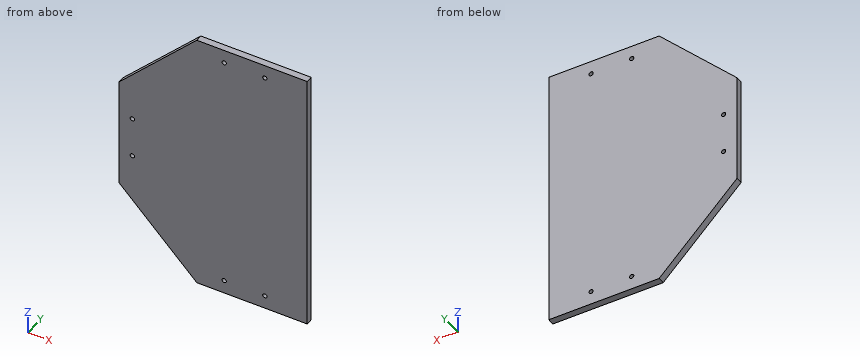
from build123d import *

# Parameters (mm, degrees)
BOSS_EXTRUDE1_DEPTH = 6.35
SKETCH2_R           = 1.995
CUT_EXTRUDE1_DEPTH  = 177.890707783
SKETCH5_R           = 1.995
CUT_EXTRUDE5_DEPTH  = 177.890707783
CUT_EXTRUDE6_DEPTH  = 10


with BuildPart() as part:
    # Sketch1 → Boss-Extrude1 (new body)
    with BuildSketch(Plane(origin=(0, 0, 0), x_dir=(1, 0, 0), z_dir=(0, 1, 0))):
        Polygon((125, 51.776695297), (51.776695297, 125), (-51.776695297, 125), (-125, 51.776695297), (-125, -51.776695297), (-51.776695297, -125), (51.776695297, -125), (125, -51.776695297), align=None)
    extrude(amount=BOSS_EXTRUDE1_DEPTH)

    # Sketch2 → Cut-Extrude1 (cut, through all)
    with BuildSketch(Plane(origin=(0, 6.35, 0), x_dir=(1, 0, 0), z_dir=(0, 1, 0))):
        with Locations(Location((-26.05, -112.3, 0), (0, 0, 270))):
            Circle(SKETCH2_R)
        with Locations(Location((12.05, -112.3, 0), (0, 0, 270))):
            Circle(SKETCH2_R)
        with Locations(Location((12.05, 112.3, 0), (0, 0, 90))):
            Circle(SKETCH2_R)
        with Locations(Location((-26.05, 112.3, 0), (0, 0, 90))):
            Circle(SKETCH2_R)
    extrude(amount=-CUT_EXTRUDE1_DEPTH, mode=Mode.SUBTRACT)

    # Sketch5 → Cut-Extrude5 (cut, through all)
    with BuildSketch(Plane(origin=(0, 6.35, 0), x_dir=(1, 0, 0), z_dir=(0, 1, 0))):
        with Locations(Location((-112.3, 19.05, 0), (0, 0, 270))):
            Circle(SKETCH5_R)
        with Locations(Location((-112.3, -19.05, 0), (0, 0, 270))):
            Circle(SKETCH5_R)
    extrude(amount=-CUT_EXTRUDE5_DEPTH, mode=Mode.SUBTRACT)

    # Sketch6 → Cut-Extrude6 (cut)
    with BuildSketch(Plane(origin=(0, 6.35, 0), x_dir=(1, 0, 0), z_dir=(0, 1, 0))):
        Polygon((51.776695297, -125), (125, -51.776695297), (125, 51.776695297), (51.776695297, 125), align=None)
    extrude(amount=-CUT_EXTRUDE6_DEPTH, mode=Mode.SUBTRACT)


solid = part.part
For this review, take the finished solid that the model builds, in its own axes (mm). Round coordinates to 2 decimals unless told otherwise and drop trailing zeros. Write each loop counter-clockwise with the first axis right and the second up, starting at its lowest first coordinate (ties: lowest second). Pieces come first, ordered by that corner, then holes. Notation, with made-up numbers: M 39,-23.75 L 71,-23.75 A20 cw 71,-7.75 Z; hole C -21.75,-8 d1. An arc over 180 degrees is marked long. Write item = value, one per line. Start each with the question number.
(1) Clearance check with flat-ended pins moving along their axes: pin 1 Ø4.5 at (x, z) = (12.05, -112.3) entering from +Y; pin 2 Ø2.5 at (x, z) = (-26.05, -112.3) entering from +Y; pin 3 Ø3 at (y, z) = (1, -73) entering from -X; pin 4 Ø3 at (y, z) = (2, -93) entering from -X. State where each tip first meets the part, or that it passes through.
(2) We need section B-B (z = 89). Give the boundary of the cut face in (x, y).
(3) We need section C-C (x = -86.5). Give the boundary of the cut face in (y, z).
(4) For line 1 along X through (y, z) = (3, -112.3) (3 decimals); line 2 along X through (y, z) = (1.5, 19.05) (3 decimals); line 3 along Z through (x, y) = (-114, 3.25), list the stretches that pass through material, from the lowest coordinate up.
(5) We need section A-A (y = 5). Give the boundary of the cut face in (x, z) (3 decimals), then the cut area to 3 significant figures.
Results found:
q1.pin_1 = 6.35
q1.pin_2 = through
q1.pin_3 = -105.28
q1.pin_4 = -85.28
q2.outline = M -87.78,0 L 51.78,0 L 51.78,6.35 L -87.78,6.35 Z
q3.outline = M 0,-90.28 L 6.35,-90.28 L 6.35,90.28 L 0,90.28 Z
q4.line_1 = -64.477 to -28.045, -24.055 to 10.055, 14.045 to 51.777
q4.line_2 = -125 to -114.295, -110.305 to 51.777
q4.line_3 = -62.78 to -20.09, -18.01 to 18.01, 20.09 to 62.78
q5.outline = M -125,-51.777 L -51.777,-125 L 51.777,-125 L 51.777,125 L -51.777,125 L -125,51.777 Z; hole C -112.3,-19.05 d3.99; hole C -112.3,19.05 d3.99; hole C -26.05,-112.3 d3.99; hole C -26.05,112.3 d3.99; hole C 12.05,-112.3 d3.99; hole C 12.05,112.3 d3.99
q5.area = 38,800 mm²
